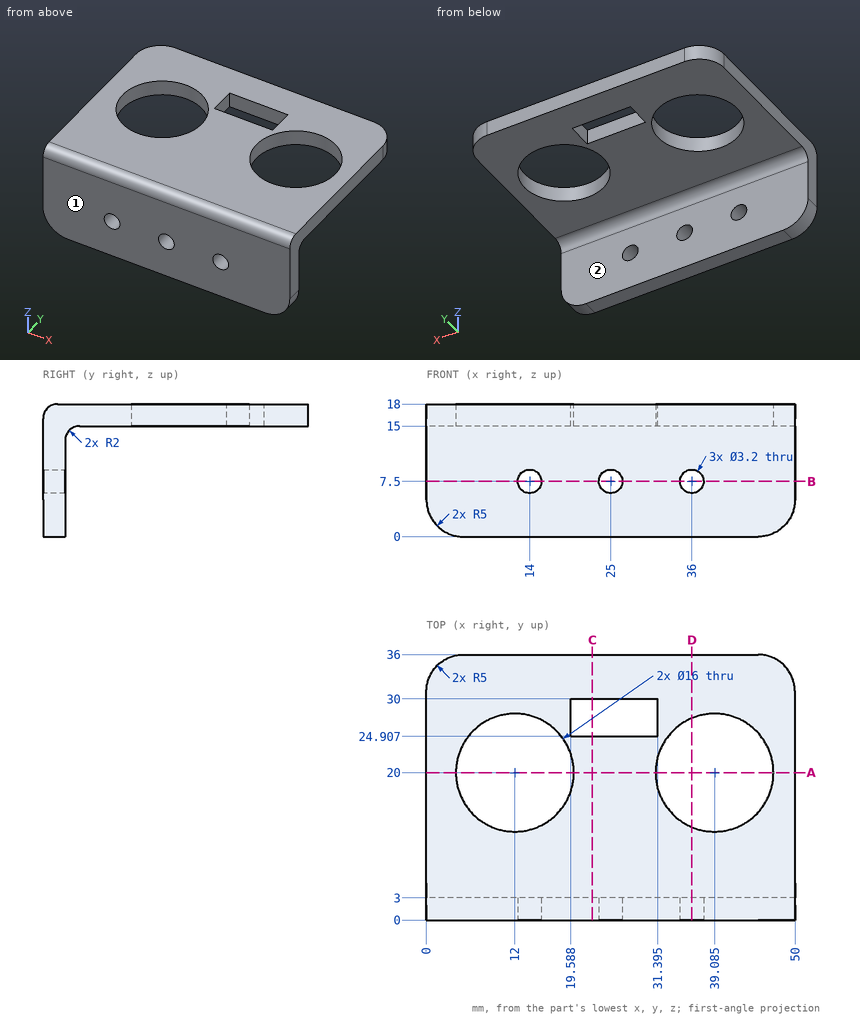
For this review, use the dimensioned drawing (mm, ordinates from the lowest corner) and the shaded views. A direction names the side the tool comes from. Round coordinates to 2 decimals unless told otherwise and drop trailing zeros. Loops run counter-clockwise (first coordinate to the right, second up) from the corner with the lowest first, then second, coordinate; pieces in that order, holes last. Notation, with made-up numbers: M 54.5,77.5 L 104.5,77.5 A22 cw 104.5,109.5 Z; hole C 31.25,-2.75 d10. An arc over 180 degrees is marked long. Answer as a JSON object with one key per item and string values.
(1) Take a section at B-B on z = 7.5. Give the boundary of the cut face in (x, y), and give its area (3 significant figures).
Resolved:
{"outline": "M 0,0 L 12.4,0 L 12.4,3 L 0,3 Z; M 15.6,0 L 23.4,0 L 23.4,3 L 15.6,3 Z; M 26.6,0 L 34.4,0 L 34.4,3 L 26.6,3 Z; M 37.6,0 L 50,0 L 50,3 L 37.6,3 Z", "area": "121 mm²"}
(2) Take a section at C-C on x = 22.5. Give the boundary of the cut face in (y, z).
Resolved:
{"outline": "M 0,0 L 3,0 L 3,13 A2 cw 5,15 L 24.91,15 L 24.91,18 L 2,18 A2 ccw 0,16 Z; M 30,15 L 36,15 L 36,18 L 30,18 Z"}
(3) To check wall thickness, follow line 1 along X through (y, z) = (2.4, 7.5); line 2 along Y through (x, z) = (12, 15.9); line 3 along X through (y, z) = (20.5, 15.25) (1 decimal). State the ranges of each line that lie inside material, in increasing order.
Resolved:
{"line 1": "0 to 12.4, 15.6 to 23.4, 26.6 to 34.4, 37.6 to 50", "line 2": "0 to 12, 28 to 36", "line 3": "0 to 4, 20 to 31.1, 47.1 to 50"}
(4) Take a section at A-A on y = 20. Give the boundary of the cut face in (x, z) (1 decimal), and give its area (3 significant figures).
Resolved:
{"outline": "M 0,15 L 4,15 L 4,18 L 0,18 Z; M 20,15 L 31.1,15 L 31.1,18 L 20,18 Z; M 47.1,15 L 50,15 L 50,18 L 47.1,18 Z", "area": "54.0 mm²"}
(5) Clearance check with a flat-ended pin moving along its axis: P1, Ø5, axis at x = 36, z = 7.5, coming from the +Y side. State where the tip first meets the part, or that it passes through.
Resolved:
{"P1": "y = 3"}
(6) Take a section at D-D on x = 36. Give the boundary of the cut face in (y, z).
Resolved:
{"outline": "M 0,0 L 3,0 L 3,5.9 L 0,5.9 Z; M 0,9.1 L 3,9.1 L 3,13 A2 cw 5,15 L 12.62,15 L 12.62,18 L 2,18 A2 ccw 0,16 Z; M 27.38,15 L 36,15 L 36,18 L 27.38,18 Z"}
(7) Tool access review of the marked faces 1 and 2: name each direction out of +Z, -Z, +X, -X, +Y, -Y from which nothing blocks a thin tool from reaching the whole face with its end or side.
Resolved:
{"face 1": "+Z, -Z, +X, -X, -Y", "face 2": "-Z, +X, -X, +Y"}
